```python
from build123d import *

# Parameters (mm, degrees)
EXTRUDE_1_DEPTH        = 25
CUT_EXTRUDE_START      = -6
CUT_EXTRUDE_2_DEPTH    = 6
PATTERN_LINEAR_1_COUNT = 2
PATTERN_LINEAR_1_PITCH = 350
MIRROR_START           = -6
MIRROR_1_COPY_1_DEPTH  = 6
CUT_EXTRUDE_3_DEPTH    = 6


with BuildPart() as part:
    # 草图1 → 凸台-拉伸1 (new body)
    with BuildSketch(Plane(origin=(0, 0, 0), x_dir=(1, 0, 0), z_dir=(0, 1, 0))):
        Polygon((0, 0), (0, -14), (50, -14), (50, -34), (0, -34), (0, -48), (898, -48), (850, 0), align=None)
    extrude(amount=EXTRUDE_1_DEPTH)

    # 草图5 → 切除-拉伸2 (cut)
    with BuildSketch(Plane(origin=(0, 25, 0), x_dir=(1, 0, 0), z_dir=(0, 1, 0)).offset(CUT_EXTRUDE_START)):
        Polygon((147.5, 0), (155, -7.5), (195, -7.5), (202.5, 0), align=None)
    cut_extrude_2 = extrude(amount=-CUT_EXTRUDE_2_DEPTH, mode=Mode.SUBTRACT)

    # 阵列(线性)1: 切除-拉伸2 ×2
    with Locations(*[(i * PATTERN_LINEAR_1_PITCH, 0, 0) for i in range(1, PATTERN_LINEAR_1_COUNT)]):
        add(cut_extrude_2, mode=Mode.SUBTRACT)

    # 镜向1: 切除-拉伸2 across plane
    add(cut_extrude_2.mirror(Plane.XY.offset(24)), mode=Mode.SUBTRACT)

    # 镜向1 copy 1 sketch → 镜向1 copy 1 (cut)
    with BuildSketch(Plane(origin=(350, 25, 48), x_dir=(1, 0, 0), z_dir=(0, 1, 0)).offset(MIRROR_START)):
        Polygon((147.5, 0), (155, 7.5), (195, 7.5), (202.5, 0), align=None)
    extrude(amount=-MIRROR_1_COPY_1_DEPTH, mode=Mode.SUBTRACT)

    # 草图6 → 切除-拉伸3 (cut)
    with BuildSketch(Plane(origin=(0, 25, 0), x_dir=(1, 0, 0), z_dir=(0, 1, 0)).offset(CUT_EXTRUDE_START)):
        Polygon((890.5, -40.5), (823, -40.5), (815.5, -48), (898, -48), align=None)
    cut_extrude_3 = extrude(amount=-CUT_EXTRUDE_3_DEPTH, mode=Mode.SUBTRACT)

    # 镜向2: 切除-拉伸3 across plane
    add(cut_extrude_3.mirror(Plane.XY.offset(24)), mode=Mode.SUBTRACT)


solid = part.part
```
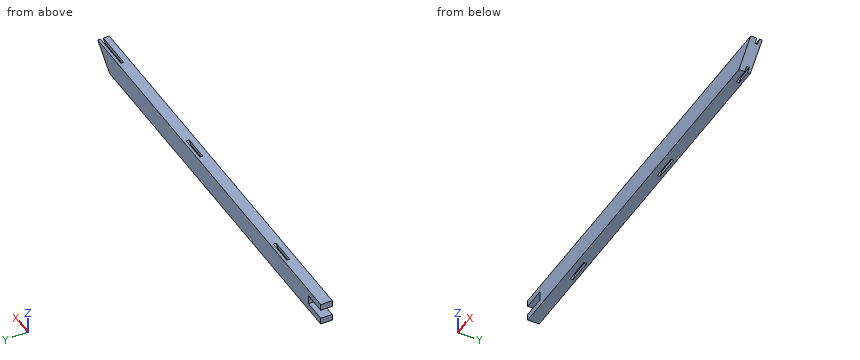
Source: CAD feature listing. Evaluate the final solid. Frame: model axes, mm. Coordinates: 2 decimals unless noted, no trailing zeros. Write each loop counter-clockwise with the first axis right and the second up, starting at its lowest first coordinate (ties: lowest second). Pieces come first, ordered by that corner, then holes. Notation, with made-up numbers: (-6.5, 2) -> (26.5, 2) arc R27 cw to (26.5, 19) -> close; hole circle Ø4 at (-39.75, 32). An arc over 180 degrees is marked (long way). Return JSON: item names as keys, results as strings. Group by question number.
1) Contact query for flat-ended pins moving along their axis: P1, Ø5, axis at x = 517.5, y = 16, coming from the -Z side; P2, Ø6, axis at y = 18.5, z = 39.5, coming from the +X side; P3, Ø10, axis at y = 6.5, z = 9, coming from the +X side. Output: stop coordinate, or through.
2) Ray query, line 1 along X through (y, z) = (14.25, 45); line 2 along X through (y, z) = (7, 23.5); line 3 along X through (y, z) = (22, 36.5). Return the intervals inside material, ascending.
3) Section query A-A, the plane y = 4.25. Return loops of the section in (x, z), plus the area to 3 significant figures.
4) Section query B-B, the plane x = 834. Return loops of the section in (y, z), plus the area to 3 significant figures.
From the geometry:
{
 "1": {"P1": "z = 7.5", "P2": "x = 892.46", "P3": "x = 864"},
 "2": {"line 1": "0 to 150.5, 199.5 to 500.5, 549.5 to 818.5", "line 2": "50 to 873.5", "line 3": "0 to 886.5"},
 "3": {"outline": "(0, 0) -> (850, 0) -> (898, 48) -> (0, 48) -> (0, 34) -> (50, 34) -> (50, 14) -> (0, 14) -> close", "area": "41,000 mm²"},
 "4": {"outline": "(0, 0) -> (13, 0) -> (13, 7.5) -> (19, 7.5) -> (19, 0) -> (25, 0) -> (25, 48) -> (19, 48) -> (19, 40.5) -> (13, 40.5) -> (13, 48) -> (0, 48) -> close", "area": "1,110 mm²"}
}
